Study the drawing (mm; zero at the part's minimum x, y, z) and answer. A direction names the side the tool comes from. Coordinates: 2 decimals unless noted, no trailing zeros. Order: outer loops, then holes, each group sorted by start corner. A loop starts at its lowest first (then second) coordinate and runs counter-clockwise, first axis right, second up.
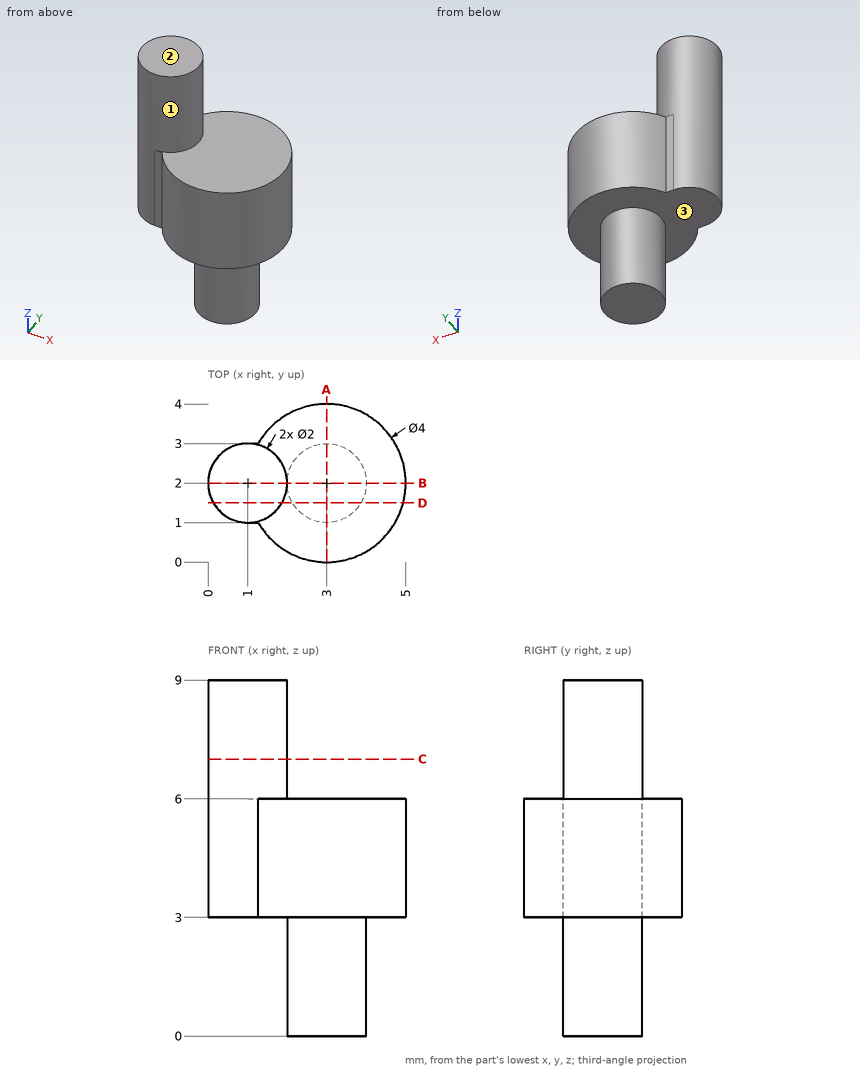
1) A cutting plane is placed at A-A, the plane x = 3. Determine the outline of the cut face in (y, z), and give its area (3 significant figures).
A:
outline: (0, 3) - (1, 3) - (1, 0) - (3, 0) - (3, 3) - (4, 3) - (4, 6) - (0, 6) - close
area: 18.0 mm2
2) Straight lines are drawn through the part: line 1 (Z direction, x = 3.65, y = 3.8); line 2 (X direction, y = 2.05, z = 8.75); line 3 (Z direction, x = 3.25, y = 1.7). For each, find the intervals that lie inside material, in ascending order.
A:
line 1: z = 3 to 6
line 2: x = 0 to 2
line 3: z = 0 to 6
3) Which of the six approach directions +Z, -Z, +X, -X, +Y, -Y give full straight-line access (tool end or side, diameter ignored) to the marked faces 1, 2 and 3?
A:
face 1: +Z
face 2: +Z, +X, -X, +Y, -Y
face 3: -Z
4) A cutting plane is placed at C-C, the plane z = 7. Determine the outline of the cut face in (x, y), and give its area (3 significant figures).
A:
outline: circle Ø2 at (1, 2)
area: 3.14 mm2
5) A cutting plane is placed at B-B, the plane y = 2. Determine the outline of the cut face in (x, z).
A:
outline: (0, 3) - (2, 3) - (2, 0) - (4, 0) - (4, 3) - (5, 3) - (5, 6) - (2, 6) - (2, 9) - (0, 9) - close
6) Flat-ended cylindrical pins translate along their axes: pin 1 Ø2 at (y, z) = (3.5, 2.5) entering from -X; pin 2 Ø1.5 at (y, z) = (3.5, 6.5) entering from +X; pin 3 Ø2 at (x, y) = (3.5, 2.5) entering from +Z. Find the tip coordinate at first contact, or state that the pin passes through.
A:
pin 1: stops at x = 0.23
pin 2: stops at x = 4.76
pin 3: stops at z = 6
7) A cutting plane is placed at D-D, the plane y = 1.5. Determine the outline of the cut face in (x, z).
A:
outline: (0.13, 3) - (2.13, 3) - (2.13, 0) - (3.87, 0) - (3.87, 3) - (4.94, 3) - (4.94, 6) - (1.87, 6) - (1.87, 9) - (0.13, 9) - close
